Print and shaded views of the part. All mm, measured from the part's lowest x, y and z. Give positions to 0.01 mm unless a question says otherwise; leave off trailing zeros. Write each loop counter-clockwise with the first axis right and the second up, starting at its lowest first coordinate (ties: lowest second). Pieces come first, ordered by that corner, then holes. Notation, with made-up numbers: M 87.5,36.5 L 98.5,36.5 A21 cw 98.5,48.5 Z; hole C -35,36 d9. An arc over 180 degrees is marked long. One line per question, with ' | ' between items. Start each with the question number.
1. Wall check: L1, parallel to X at y = 2.45, z = 169; L2, parallel to Z at x = 61, y = 2.5. Give the ranges that are in metal, low to high.
2. Flat gauge pins, fed straight in: pin 1 (3 mm diameter, centred on x = 98.5, y = 2, fed in from +Z); pin 2 (3 mm diameter, centred on y = 1.5, z = 80, fed in from +X); pin 3 (3 mm diameter, centred on y = 4, z = 88, fed in from -X). Where does each tip first touch, or does it go through?
3. Cut at A-A, the plane z = 90.5. Write the cut outline in (x, y), then the cut area to 3 significant figures.
4. Cut at B-B, the plane x = 70. Write the cut outline in (y, z), then the cut area to 3 significant figures.
5. Cut at C-C, the plane y = 4.55. Count the separate pieces of the cut face and the enclosed holes in it, then the cut area to 3 significant figures.
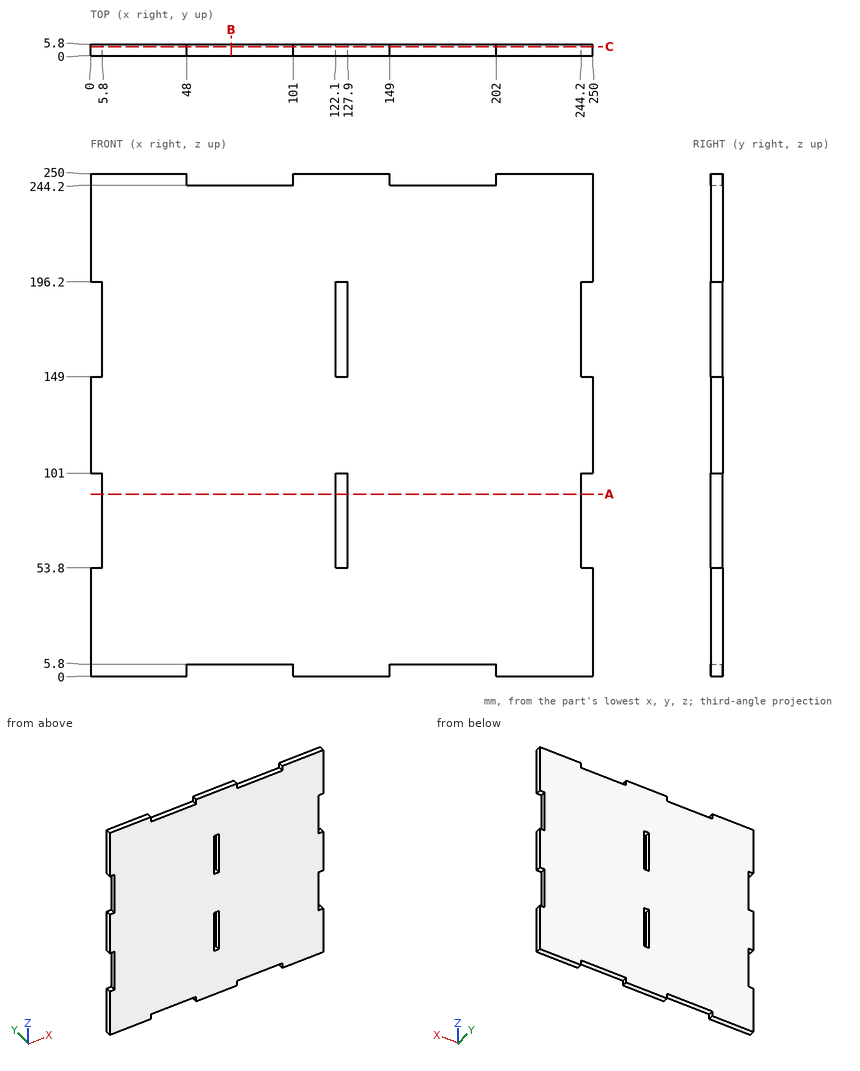
Here are the results:
1) L1: 5.8 to 122.1, 127.9 to 244.2 | L2: 5.8 to 244.2
2) pin 1: z = 244.2 | pin 2: x = 244.2 | pin 3: x = 5.8
3) outline: M 5.8,0 L 122.1,0 L 122.1,5.8 L 5.8,5.8 Z; M 127.9,0 L 244.2,0 L 244.2,5.8 L 127.9,5.8 Z | area: 1,350 mm^2
4) outline: M 0,5.8 L 5.8,5.8 L 5.8,244.2 L 0,244.2 Z | area: 1,380 mm^2
5) separate pieces: 1 | enclosed holes: 2 | area: 59,600 mm^2
